Read the model definition and answer for the solid it produces. Units are mm, in the model's axes. Give positions to 0.01 mm unless a question says otherwise; leave off trailing zeros. Order: outer loops, then holes, each group sorted by start corner. A loop starts at its lowest first (then second) coordinate and runs counter-clockwise, first axis right, second up. Notation, with made-up numbers: (34, 44.25) -> (84, 44.25) arc R15 ccw to (84, 53.25) -> close; hole circle Ø1 at (14, 1). An arc over 180 degrees is marked (long way). Answer as CSV lines item,"result". Start each with the question number.
1) Find section C-C (y = 2.75). Determine the outline of the cut face in (x, z).
2) Flat-ended cylindrical pins translate along their axes: pin 1 Ø1.5 at (x, y) = (2, 1) entering from +Z; pin 2 Ø2 at (y, z) = (5.5, 2) entering from +X; pin 3 Ø2 at (x, y) = (3, 5.5) entering from -Z. Find the tip coordinate at first contact, or state that the pin passes through.
3) Find section B-B (x = 0). Determine the outline of the cut face in (y, z).
4) The mould has two halves that part along Z. Classify faces 1 (the face through (-3.905, 3.458, -0.867)), 2 (the face through (0, 1, 0)), 3 (the face through (0, 0, 0)): +Z half, -Z half, draft (parallel to the pull), parting line (faces both ways), or undercut.
5) Straight lines are drawn through the part: L1, parallel to X at y = 3.3, z = 0; L2, parallel to Y at x = 0.75, z = 2; L3, parallel to X at y = 2, z = -0.75. For each, find the intervals that lie inside material, in ascending order. Write a range as from..to.
6) Find section A-A (z = 0). Determine the outline of the cut face in (x, y).
```python
from build123d import *

# Parameters (mm, degrees)
SKETCH1_R           = 4
BOSS_EXTRUDE1_DEPTH = 7
SKETCH2_R           = 3.05
CUT_EXTRUDE1_DEPTH  = 6
CHAMFER1_SIZE       = 0.5


with BuildPart() as part:
    # Sketch1 → Boss-Extrude1 (new body)
    with BuildSketch(Plane(origin=(0, 0, 0), x_dir=(1, 0, 0), z_dir=(0, 1, 0))):
        with Locations(Location((0, 0, 0), (0, 0, 270))):
            Circle(SKETCH1_R)
    extrude(amount=BOSS_EXTRUDE1_DEPTH)

    # Sketch2 → Cut-Extrude1 (cut)
    with BuildSketch(Plane(origin=(0, 7, 0), x_dir=(1, 0, 0), z_dir=(0, 1, 0))):
        with Locations(Location((0, 0, 0), (0, 0, 270))):
            Circle(SKETCH2_R)
    extrude(amount=-CUT_EXTRUDE1_DEPTH, mode=Mode.SUBTRACT)

    # Chamfer1
    chamfer1_edges = [part.edges().sort_by_distance(p)[0] for p in [
        (0, 0, -4),
        (0, 7, -4),
    ]]
    chamfer(chamfer1_edges, length=CHAMFER1_SIZE)


solid = part.part
```
Findings below:
1,outline,"circle Ø8 at (0, 0); hole circle Ø6.1 at (0, 0)"
2,pin 1,"z = 3.8"
2,pin 2,"x = 3.87"
2,pin 3,"z = -3.46"
3,outline,"(0, -3.5) -> (0.5, -4) -> (6.5, -4) -> (7, -3.5) -> (7, -3.05) -> (1, -3.05) -> (1, 3.05) -> (7, 3.05) -> (7, 3.5) -> (6.5, 4) -> (0.5, 4) -> (0, 3.5) -> close"
4,face 1,"parting line"
4,face 2,"undercut"
4,face 3,"draft"
5,L1,"-4..-3.05, 3.05..4"
5,L2,"0..1"
5,L3,"-3.93..-2.96, 2.96..3.93"
6,outline,"(-4, 0.5) -> (-3.5, 0) -> (3.5, 0) -> (4, 0.5) -> (4, 6.5) -> (3.5, 7) -> (3.05, 7) -> (3.05, 1) -> (-3.05, 1) -> (-3.05, 7) -> (-3.5, 7) -> (-4, 6.5) -> close"
